Geometry check sheet. Reference: the model listing, model coordinates, mm. Round coordinates to 2 decimals unless told otherwise and drop trailing zeros. Write each loop counter-clockwise with the first axis right and the second up, starting at its lowest first coordinate (ties: lowest second). Pieces come first, ordered by that corner, then holes. Notation, with made-up numbers: (57, -10.75) - (116, -10.75) arc R22 cw to (116, 26.25) - close; hole circle Ø10 at (10.25, 26.5). An arc over 180 degrees is marked (long way). One line per question, with ' | ' between items. Start each with the question number.
from build123d import *

# Parameters (mm, degrees)
SKETCH1_W            = 40
SKETCH1_H            = 39
BOSS_EXTRUDE1_DEPTH  = 1.5
SKETCH3_W            = 70
SKETCH3_H            = 49
BOSS_EXTRUDE2_DEPTH  = 1.5
SKETCH4_W            = 13
SKETCH4_H            = 12
CUT_EXTRUDE1_DEPTH   = 52.259145525
SKETCH5_W            = 15.6
SKETCH5_H            = 15.6
CUT_EXTRUDE2_DEPTH   = 52.259145525
FILLET2_R            = 2
SKETCH6_R            = 1.1
CUT_EXTRUDE3_DEPTH   = 52.259145525
FILLET4_R            = 2.5
SKETCH7_W            = 14
SKETCH7_H            = 14
CUT_EXTRUDE4_DEPTH   = 52.259145525
LPATTERN1_COUNT      = 2
LPATTERN1_PITCH      = 19
LPATTERN1_COUNT_DIR2 = 2
LPATTERN1_PITCH_DIR2 = 19
FILLET5_R            = 2


with BuildPart() as part:
    # Sketch1 → Boss-Extrude1 (new body)
    with BuildSketch(Plane(origin=(0, 0, 0), x_dir=(1, 0, 0), z_dir=(0, 1, 0))):
        Rectangle(SKETCH1_W, SKETCH1_H)
    extrude(amount=BOSS_EXTRUDE1_DEPTH)

    # Sketch3 → Boss-Extrude2 (add)
    with BuildSketch(Plane(origin=(0, 0, 0), x_dir=(1, 0, 0), z_dir=(0, 1, 0))):
        with Locations((-10, 0)):
            Rectangle(SKETCH3_W, SKETCH3_H)
    extrude(amount=BOSS_EXTRUDE2_DEPTH)

    # Sketch4 → Cut-Extrude1 (cut, through all)
    with BuildSketch(Plane(origin=(0, 1.5, 0), x_dir=(1, 0, 0), z_dir=(0, 1, 0))):
        with Locations((-38.5, 8.5)):
            Rectangle(SKETCH4_W, SKETCH4_H)
    extrude(amount=-CUT_EXTRUDE1_DEPTH, mode=Mode.SUBTRACT)

    # Sketch5 → Cut-Extrude2 (cut, through all)
    with BuildSketch(Plane(origin=(0, 1.5, 0), x_dir=(1, 0, 0), z_dir=(0, 1, 0))):
        with Locations((-29.2, -9.5)):
            Rectangle(SKETCH5_W, SKETCH5_H)
    extrude(amount=-CUT_EXTRUDE2_DEPTH, mode=Mode.SUBTRACT)

    # Fillet2
    fillet2_edges = [part.edges().sort_by_distance(p)[0] for p in [
        (-37, 0.75, 17.3),
        (-37, 0.75, 1.7),
        (-21.4, 0.75, 1.7),
        (-21.4, 0.75, 17.3),
    ]]
    fillet(fillet2_edges, radius=FILLET2_R)

    # Sketch6 → Cut-Extrude3 (cut, through all)
    with BuildSketch(Plane(origin=(0, 1.5, 0), x_dir=(1, 0, 0), z_dir=(0, 1, 0))):
        with Locations(Location((-41.75, 21.25, 0), (0, 0, 270))):
            Circle(SKETCH6_R)
        with Locations(Location((21.75, 21.25, 0), (0, 0, 270))):
            Circle(SKETCH6_R)
        with Locations(Location((21.75, -21.25, 0), (0, 0, 270))):
            Circle(SKETCH6_R)
        with Locations(Location((-41.75, -21.25, 0), (0, 0, 270))):
            Circle(SKETCH6_R)
        with Locations(Location((-10, -21.25, 0), (0, 0, 270))):
            Circle(SKETCH6_R)
        with Locations(Location((-10, 21.25, 0), (0, 0, 270))):
            Circle(SKETCH6_R)
    extrude(amount=-CUT_EXTRUDE3_DEPTH, mode=Mode.SUBTRACT)

    # Fillet4
    fillet4_edges = [part.edges().sort_by_distance(p)[0] for p in [
        (25, 0.75, 24.5),
        (25, 0.75, -24.5),
        (-45, 0.75, -24.5),
        (-45, 0.75, 24.5),
        (-45, 0.75, -2.5),
        (-45, 0.75, -14.5),
    ]]
    fillet(fillet4_edges, radius=FILLET4_R)

    # Sketch7 → Cut-Extrude4 (cut, through all)
    with BuildSketch(Plane(origin=(0, 1.5, 0), x_dir=(1, 0, 0), z_dir=(0, 1, 0))):
        with Locations((-9, 9.5)):
            Rectangle(SKETCH7_W, SKETCH7_H)
    cut_extrude4 = extrude(amount=-CUT_EXTRUDE4_DEPTH, mode=Mode.SUBTRACT)

    # LPattern1: Cut-Extrude4 2 × 2
    with Locations(*[(i * LPATTERN1_PITCH, 0, j * LPATTERN1_PITCH_DIR2) for i in range(LPATTERN1_COUNT) for j in range(LPATTERN1_COUNT_DIR2) if (i, j) != (0, 0)]):
        add(cut_extrude4, mode=Mode.SUBTRACT)

    # Fillet5
    fillet5_edges = [part.edges().sort_by_distance(p)[0] for p in [
        (-32, 0.75, -14.5),
        (-32, 0.75, -2.5),
    ]]
    fillet(fillet5_edges, radius=FILLET5_R)


solid = part.part
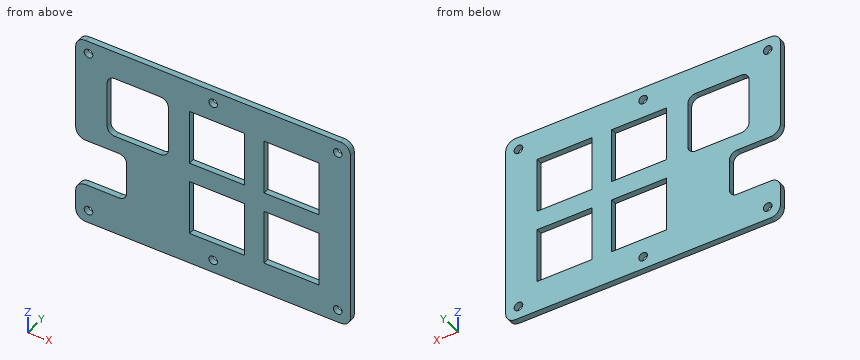
Q1. Section check B-B, the plane z = -21.25. Record the cut outline in (x, y).
Q2. Section check C-C, the plane x = -41.75. Record the cut outline in (y, z), then the cut area to 3 significant figures.
Q3. Section check D-D, the plane x = 21.75. Record the cut outline in (y, z), then the cut area to 3 significant figures.
Q4. Section check A-A, the plane x = -10. Record the cut outline in (y, z).
Q5. Thickness scan on line 1 (X direction, y = 0.5, z = -21.25); line 2 (Z direction, x = -7, y = 0.95); line 3 (X direction, y = 0.3, z = -9.5). Record the ranges inside material, lowest first.
Result sheet:
1) outline: (-45, 0) - (-42.85, 0) - (-42.85, 1.5) - (-45, 1.5) - close; (-40.65, 0) - (-11.1, 0) - (-11.1, 1.5) - (-40.65, 1.5) - close; (-8.9, 0) - (20.65, 0) - (20.65, 1.5) - (-8.9, 1.5) - close; (22.85, 0) - (25, 0) - (25, 1.5) - (22.85, 1.5) - close
2) outline: (0, -24.5) - (1.5, -24.5) - (1.5, -22.35) - (0, -22.35) - close; (0, -20.15) - (1.5, -20.15) - (1.5, -14.5) - (0, -14.5) - close; (0, -2.5) - (1.5, -2.5) - (1.5, 20.15) - (0, 20.15) - close; (0, 22.35) - (1.5, 22.35) - (1.5, 24.5) - (0, 24.5) - close | area: 48.9 mm²
3) outline: (0, -24.5) - (1.5, -24.5) - (1.5, -22.35) - (0, -22.35) - close; (0, -20.15) - (1.5, -20.15) - (1.5, 20.15) - (0, 20.15) - close; (0, 22.35) - (1.5, 22.35) - (1.5, 24.5) - (0, 24.5) - close | area: 66.9 mm²
4) outline: (0, -24.5) - (1.5, -24.5) - (1.5, -22.35) - (0, -22.35) - close; (0, -20.15) - (1.5, -20.15) - (1.5, -16.5) - (0, -16.5) - close; (0, -2.5) - (1.5, -2.5) - (1.5, 2.5) - (0, 2.5) - close; (0, 16.5) - (1.5, 16.5) - (1.5, 20.15) - (0, 20.15) - close; (0, 22.35) - (1.5, 22.35) - (1.5, 24.5) - (0, 24.5) - close
5) line 1: -45 to -42.85, -40.65 to -11.1, -8.9 to 20.65, 22.85 to 25 | line 2: -24.5 to -16.5, -2.5 to 2.5, 16.5 to 24.5 | line 3: -32 to -16, -2 to 3, 17 to 25
